Geometry check sheet. Reference: the model listing, model coordinates, mm. Face numbers are marked on the shaded views. Round coordinates to 2 decimals unless told otherwise and drop trailing zeros. Order: outer loops, then holes, each group sorted by start corner. A loop starts at its lowest first (then second) coordinate and runs counter-clockwise, first axis right, second up.
```python
from build123d import *

# Parameters (mm, degrees)
SKETCH1_R               = 65
BOSS_EXTRUDE1_DEPTH     = 10
CUT_EXTRUDE4_DEPTH      = 93.466210045
CUT_EXTRUDE4_DEPTH_BACK = 93.466210045
SKETCH2_OUTSIDE_W       = 168.824
SKETCH2_OUTSIDE_H       = 168.824
SKETCH3_R               = 7.5
CUT_EXTRUDE5_DEPTH      = 10


with BuildPart() as part:
    # Sketch1 → Boss-Extrude1 (new body)
    with BuildSketch(Plane.XY):
        Circle(SKETCH1_R)
    extrude(amount=BOSS_EXTRUDE1_DEPTH)

    # Sketch2 outside → Cut-Extrude4 (cut, two sides: drawn at the far end of the back side and taken through both)
    with BuildSketch(Plane(origin=(0, 0, 0), x_dir=(-1, 0, 0), z_dir=(0, 0, -1)).offset(-CUT_EXTRUDE4_DEPTH_BACK)):
        Rectangle(SKETCH2_OUTSIDE_W, SKETCH2_OUTSIDE_H)
        with BuildLine():
            ThreePointArc((-5.730851082, 64.746871321), (-11.623493415, 63.952282217), (-17.418870891, 62.62254336))
            ThreePointArc((-17.418870891, 62.62254336), (-21.592454328, 52.644679623), (-31.570318066, 56.818263061))
            ThreePointArc((-31.570318066, 56.818263061), (-36.630326198, 53.695616233), (-41.383813447, 50.123646961))
            ThreePointArc((-41.383813447, 50.123646961), (-41.138208837, 39.310865549), (-51.950990248, 39.065260939))
            ThreePointArc((-51.950990248, 39.065260939), (-55.303442804, 34.154490393), (-58.193118697, 28.957916642))
            ThreePointArc((-58.193118697, 28.957916642), (-53.570793308, 19.179845694), (-63.348864256, 14.557520305))
            ThreePointArc((-63.348864256, 14.557520305), (-64.414091734, 8.707742879), (-64.940305058, 2.785099462))
            ThreePointArc((-64.940305058, 2.785099462), (-56.740500941, -4.267543725), (-63.793144129, -12.467347841))
            ThreePointArc((-63.793144129, -12.467347841), (-62.38695902, -18.244652485), (-60.458722709, -23.869286717))
            ThreePointArc((-60.458722709, -23.869286717), (-50.099260491, -26.977036065), (-53.207009838, -37.336498283))
            ThreePointArc((-53.207009838, -37.336498283), (-49.572554323, -42.042381687), (-45.523277954, -46.396456377))
            ThreePointArc((-45.523277954, -46.396456377), (-34.795402763, -45.02195379), (-33.420900177, -55.749828981))
            ThreePointArc((-33.420900177, -55.749828981), (-28.186604631, -58.570601153), (-22.716444875, -60.90125723))
            ThreePointArc((-22.716444875, -60.90125723), (-13.475103792, -55.282166693), (-7.856013255, -64.523507776))
            ThreePointArc((-7.856013255, -64.523507776), (-1.926934931, -64.971431582), (4.018267896, -64.875677439))
            ThreePointArc((4.018267896, -64.875677439), (10.175163042, -55.983590753), (19.067249728, -62.140485899))
            ThreePointArc((19.067249728, -62.140485899), (24.665919324, -60.138111243), (30.058185642, -57.632503641))
            ThreePointArc((30.058185642, -57.632503641), (32.066051748, -47.004943376), (42.693612013, -49.012809482))
            ThreePointArc((42.693612013, -49.012809482), (46.993812045, -44.906365133), (50.900770021, -40.424146388))
            ThreePointArc((50.900770021, -40.424146388), (48.412428796, -29.898714263), (58.937860921, -27.410373038))
            ThreePointArc((58.937860921, -27.410373038), (61.196047738, -21.90990053), (62.942148845, -16.226086984))
            ThreePointArc((62.942148845, -16.226086984), (56.387857092, -7.622725833), (64.991218242, -1.06843408))
            ThreePointArc((64.991218242, -1.06843408), (64.816930829, 4.87498492), (64.100258321, 10.77761027))
            ThreePointArc((64.100258321, 10.77761027), (54.613312629, 15.971301144), (59.807003503, 25.458246837))
            ThreePointArc((59.807003503, 25.458246837), (57.230377735, 30.816941189), (54.174850802, 35.917760796))
            ThreePointArc((54.174850802, 35.917760796), (43.395630266, 36.803745059), (44.281614528, 47.582965594))
            ThreePointArc((44.281614528, 47.582965594), (39.74817241, 51.430368364), (34.882119415, 54.847404178))
            ThreePointArc((34.882119415, 54.847404178), (24.674449193, 51.272487101), (21.099532116, 61.480157323))
            ThreePointArc((21.099532116, 61.480157323), (15.393146975, 63.151017618), (9.557952688, 64.293433105))
            ThreePointArc((9.557952688, 64.293433105), (1.686831695, 56.875750328), (-5.730851082, 64.746871321))
        make_face(mode=Mode.SUBTRACT)
    extrude(amount=CUT_EXTRUDE4_DEPTH + CUT_EXTRUDE4_DEPTH_BACK, mode=Mode.SUBTRACT)

    # Sketch3 → Cut-Extrude5 (cut)
    with BuildSketch(Plane.XY.offset(10)):
        Circle(SKETCH3_R)
    extrude(amount=-CUT_EXTRUDE5_DEPTH, mode=Mode.SUBTRACT)


solid = part.part
```
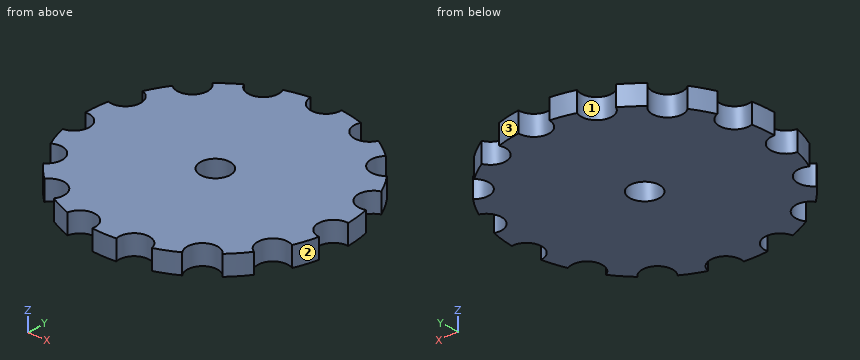
(1) Draft check along Y on the marked faces 1, 2 and 3. Enter one of: released by +Y, released by -Y, zero draft, split by the parting line, or undercut.
Returned:
face 1: undercut
face 2: released by -Y
face 3: released by +Y
(2) Sectioned sample at C-C, the plane x = 24.5. Record the cut outline in (y, z), and give its area (3 significant figures).
Returned:
outline: (-60.21, 0) - (52.07, 0) - (52.07, 10) - (-60.21, 10) - close
area: 1,120 mm2
(3) Depth check by flat-ended pin: P1, Ø1.5, axis at y = 48.5, z = 2, coming from the +X side; P2, Ø1, axis at y = -27, z = 6, coming from the +X side. Enter the tip coordinate at first touch or a pass-through.
Returned:
P1: stops at x = 40.6
P2: stops at x = 50.38
(4) Sectioned sample at A-A, the plane x = 0. Record the cut outline in (y, z), and give its area (3 significant figures).
Returned:
outline: (-65, 0) - (-7.5, 0) - (-7.5, 10) - (-65, 10) - close; (7.5, 0) - (57.12, 0) - (57.12, 10) - (7.5, 10) - close
area: 1,070 mm2
(5) Material ranges on line 1 (Y direction, x = -1.5, z = 7.75); line 2 (X direction, y = -5, z = 6); line 3 (Y direction, x = 0, z = 3), recorded low to high.
Returned:
line 1: y = -64.98 to -7.35, 7.35 to 56.88
line 2: x = -57.24 to -5.59, 5.59 to 56.72
line 3: y = -65 to -7.5, 7.5 to 57.12
(6) Sectioned sample at D-D, the plane y = 31. Record the cut outline in (x, z), and give its area (3 significant figures).
Returned:
outline: (-57.13, 0) - (57.13, 0) - (57.13, 10) - (-57.13, 10) - close
area: 1,140 mm2
